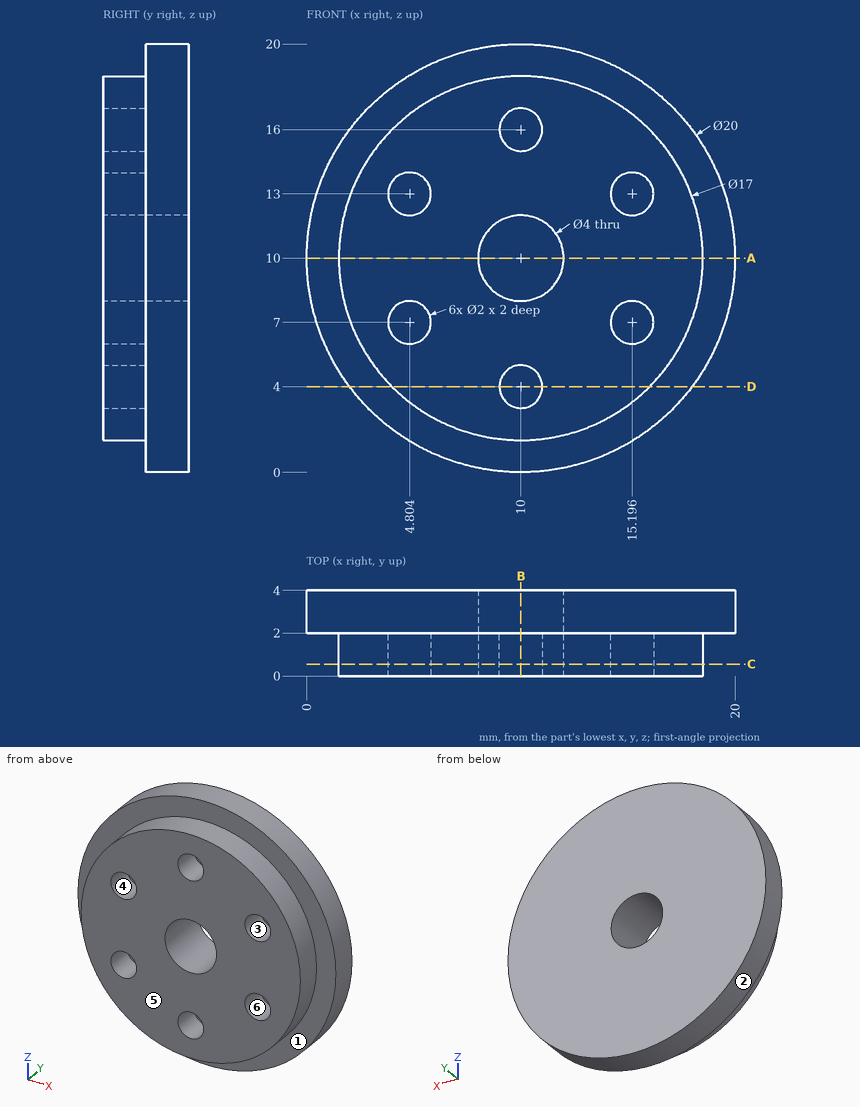
Check sheet for the drawn part. Datum: minimum x, y, z corner. Units: mm. A direction names the side the tool comes from. Round coordinates to 2 decimals unless told otherwise and drop trailing zeros. Write each loop counter-clockwise with the first axis right and the second up, starting at its lowest first coordinate (ties: lowest second). Pieces come first, ordered by that corner, then holes. Notation, with made-up numbers: (-38.5, 22.25) -> (-23.5, 22.25) arc R20 ccw to (-23.5, 41.25) -> close; hole circle Ø2 at (-26.5, 68). An arc over 180 degrees is marked (long way). Put each result on its own line as item: value.
(1) Go/stop test with flat-tipped pins: pin 1 Ø2 at (x, z) = (5, 7) entering from -Y; pin 2 Ø0.6 at (x, z) = (5, 13) entering from -Y. Record where each tip stops, or that it passes through.
Values found:
pin 1: stops at y = 0
pin 2: stops at y = 2
(2) Mould release check, pull along X, two halves, no side actions. Record for the marked faces 1, 2, 3 and 4: released by +X, released by -X, zero draft, split by the parting line, or undercut.
Values found:
face 1: zero draft
face 2: split by the parting line
face 3: undercut
face 4: undercut
(3) Sectioned sample at A-A (z = 10). Enter the section's corners in (x, y).
Values found:
outline: (0, 2) -> (1.5, 2) -> (1.5, 0) -> (8, 0) -> (8, 4) -> (0, 4) -> close; (12, 0) -> (18.5, 0) -> (18.5, 2) -> (20, 2) -> (20, 4) -> (12, 4) -> close
(4) Material ranges on line 1 (X direction, y = 0.5, z = 7.75) (1 decimal); line 2 (Z direction, x = 10, y = 2.9); line 3 (Z direction, x = 8.5, y = 3.15), recorded low to high.
Values found:
line 1: x = 1.8 to 4.1, 5.5 to 14.5, 15.9 to 18.2
line 2: z = 0 to 8, 12 to 20
line 3: z = 0.11 to 8.68, 11.32 to 19.89
(5) Sectioned sample at C-C (y = 0.55). Enter the section's corners in (x, z), plus the area to 3 significant figures.
Values found:
outline: circle Ø17 at (10, 10); hole circle Ø2 at (4.8, 7); hole circle Ø2 at (4.8, 13); hole circle Ø4 at (10, 10); hole circle Ø2 at (10, 4); hole circle Ø2 at (10, 16); hole circle Ø2 at (15.2, 7); hole circle Ø2 at (15.2, 13)
area: 196 mm^2
(6) Sectioned sample at B-B (x = 10). Enter the section's corners in (y, z).
Values found:
outline: (0, 1.5) -> (2, 1.5) -> (2, 0) -> (4, 0) -> (4, 8) -> (0, 8) -> (0, 5) -> (2, 5) -> (2, 3) -> (0, 3) -> close; (0, 12) -> (4, 12) -> (4, 20) -> (2, 20) -> (2, 18.5) -> (0, 18.5) -> (0, 17) -> (2, 17) -> (2, 15) -> (0, 15) -> close
(7) Sectioned sample at D-D (z = 4). Enter the section's corners in (x, y).
Values found:
outline: (2, 2) -> (3.98, 2) -> (3.98, 0) -> (9, 0) -> (9, 2) -> (11, 2) -> (11, 0) -> (16.02, 0) -> (16.02, 2) -> (18, 2) -> (18, 4) -> (2, 4) -> close
(8) Tool access check on the marked faces 5 and 6. Record the directions out of +Z, -Z, +X, -X, +Y, -Y that give a thin tool (end or side, any length) a straight path to the whole face; none if there is none.
Values found:
face 5: +Z, -Z, +X, -X, -Y
face 6: -Y
